Part model, mm, in its own coordinate system. Round coordinates to 2 decimals unless told otherwise and drop trailing zeros. Write each loop counter-clockwise with the first axis right and the second up, starting at its lowest first coordinate (ties: lowest second). Pieces come first, ordered by that corner, then holes. Notation, with made-up numbers: M 9.25,64.5 L 23.25,64.5 A23 ccw 23.25,86.5 Z; hole C -35,-17.5 d10. An arc over 180 degrees is marked long. Use a Markdown table: item, result. Add a question column.
1) Drop a flat-ended pin along its axis: P1, Ø2, axis at y = -54.5, z = 0, coming from the +X side. Give the stop position or say it passes through.
2) Slice it at C-C on y = -54.5. Give the number of separate pieces and of enclosed holes in the cut face, plus the area to 3 significant figures.
3) Slice it at A-A on y = 0. Write the cut outline in (x, z).
4) Slice it at B-B on x = 12.5. Write the cut outline in (y, z).
5) Wall check: probe 1 along Y at (x, z) = (15, 0.25); probe 2 along Y at (x, z) = (-20.75, -1.75); probe 3 along Z at (x, y) = (12, -27). Give the ranges that are in metal, low to high.
6) Two-plate mould, pull along Z, no slides. Class faces 1 (the face through (10.23, -54.55, 1.25)), 2 (the face through (0, 57.5, 0)), 3 (the face through (-0.43, 53.26, 0.16)), 4 (the face through (0, 1, -3)): released by +Z, released by -Z, zero draft, split by the parting line, or undercut.
```python
from build123d import *

# Parameters (mm, degrees)
SKETCH_1_W           = 61.5
SKETCH_1_H           = 115
EXTRUDE_1_DEPTH      = 3
M3X0_5_1_D           = 2.5
M3X0_5_1_ON_FACE_2_D = 2.5
M3X0_5_1_ON_FACE_3_D = 2.5


with BuildPart() as part:
    # ｽｹｯﾁ1 → ﾎﾞｽ - 押し出し1 (new, symmetric)
    with BuildSketch(Plane.XY):
        Rectangle(SKETCH_1_W, SKETCH_1_H)
    extrude(amount=EXTRUDE_1_DEPTH, both=True)

    # M3x0.5 ねじ穴1 (through all)
    with Locations(Plane(origin=(-20.75, 17.5, 3), x_dir=(1, 0, 0), z_dir=(0, 0, 1))):
        with Locations((0, 0), (20.75, 0), (41.5, 0), (41.5, -72), (20.75, -72), (0, -72)):
            Hole(M3X0_5_1_D / 2)

    # M3x0.5 ねじ穴1 on face 2 (through all)
    with Locations(Plane(origin=(30.75, 54.5, 0), x_dir=(0, 0, 1), z_dir=(1, 0, 0))):
        with Locations((0, 0), (0, 27.25), (0, 54.5), (0, 81.75), (0, 109)):
            Hole(M3X0_5_1_ON_FACE_2_D / 2)

    # M3x0.5 ねじ穴1 on face 3 (through all)
    with Locations(Plane(origin=(-30.75, -54.5, 0), x_dir=(0, 0, -1), z_dir=(-1, 0, 0))):
        with Locations((0, 0), (0, -27.25), (0, -54.5), (0, -81.75), (0, -109)):
            Hole(M3X0_5_1_ON_FACE_3_D / 2)


solid = part.part
```
Entries:
| question | item | result |
|---|---|---|
| 1 | P1 | passes through |
| 2 | separate pieces | 8 |
| 2 | enclosed holes | 0 |
| 2 | area | 189 mm^2 |
| 3 | outline | M -30.75,-3 L 30.75,-3 L 30.75,-1.25 L -30.75,-1.25 Z; M -30.75,1.25 L 30.75,1.25 L 30.75,3 L -30.75,3 Z |
| 4 | outline | M -57.5,-3 L 57.5,-3 L 57.5,3 L -57.5,3 Z; hole C -54.5,0 d2.5; hole C -27.25,0 d2.5; hole C 0,0 d2.5; hole C 27.25,0 d2.5; hole C 54.5,0 d2.5 |
| 5 | probe 1 | y = -57.5 to -55.72, -53.28 to -28.47, -26.03 to -1.22, 1.22 to 26.03, 28.47 to 53.28, 55.72 to 57.5 |
| 5 | probe 2 | y = -57.5 to -55.75, -53.25 to 16.25, 18.75 to 57.5 |
| 5 | probe 3 | z = -3 to -1.22, 1.22 to 3 |
| 6 | face 1 | undercut |
| 6 | face 2 | zero draft |
| 6 | face 3 | undercut |
| 6 | face 4 | released by -Z |
